The figure shows three views and two pictorial views of one solid part (mm, origin at its lowest corner). Answer the questions. Give positions to 0.01 mm unless a question says otherwise; leave off trailing zeros. Order: outer loops, then holes, each group sorted by start corner. A loop starts at its lowest first (then second) coordinate and runs counter-clockwise, first axis right, second up. Notation, with made-up numbers: (10.25, 27) - (59.25, 27) arc R20 ccw to (59.25, 54) - close; hole circle Ø11 at (16.5, -26.5). An arc over 180 degrees is marked (long way). Use a Markdown table: item, result. Add a question column.
1. Flat-ended cylindrical pins translate along their axes: P1, Ø6, axis at y = 4.5, z = 91.5, coming from the +X side; P2, Ø1.5, axis at y = 7.5, z = 113.5, coming from the -X side; P3, Ø1, axis at y = 4, z = 26, coming from the +X side; P4, Ø10, axis at x = 39, z = 59.5, coming from the -Y side. Find the tip coordinate at first contact, or state that the pin passes through.
2. Consider L1, parallel to X at y = 6, z = 110; L2, parallel to X at y = 1, z = 42; L3, parallel to Z at x = 35, y = 0.5. Determine where each line is inside the solid, lowest interval first.
3. A cutting plane is placed at C-C on y = 6.25. Determine the outline of the cut face in (x, z), and give its area (3 significant figures).
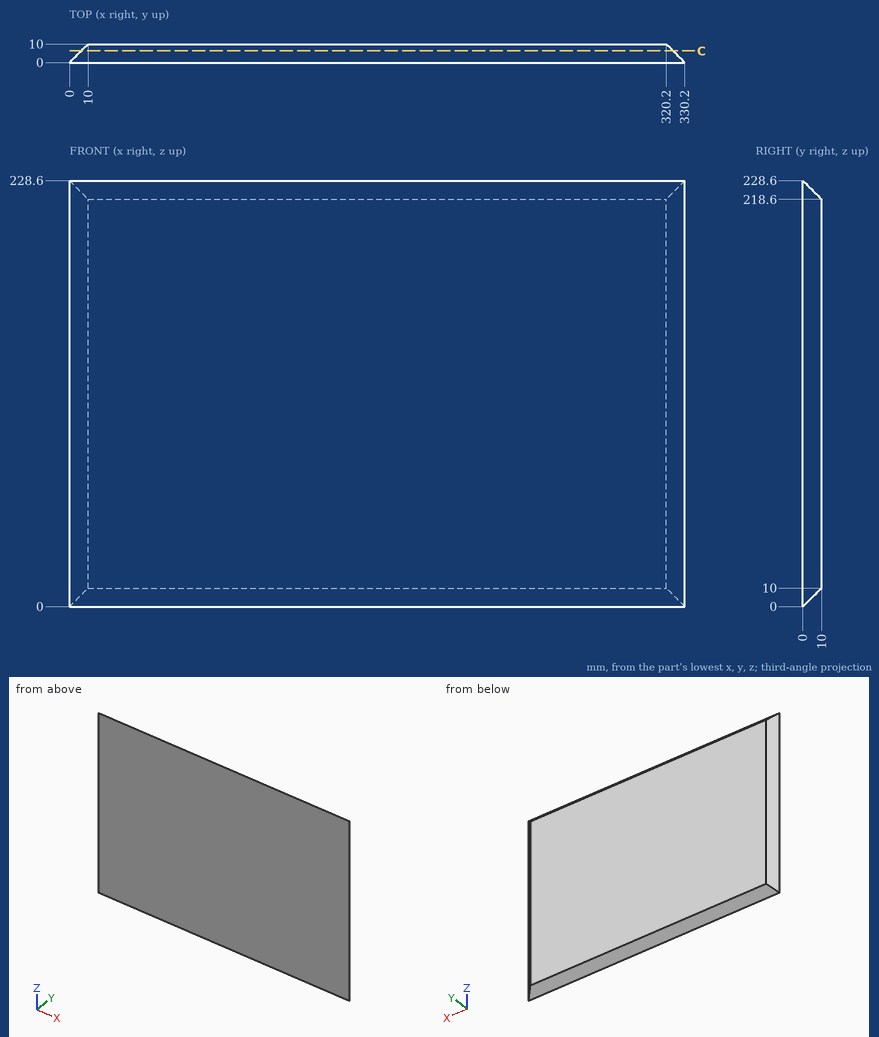
Output values:
| question | item | result |
|---|---|---|
| 1 | P1 | x = 328.7 |
| 1 | P2 | x = 6.75 |
| 1 | P3 | x = 326.7 |
| 1 | P4 | y = 0 |
| 2 | L1 | 6 to 324.2 |
| 2 | L2 | 1 to 329.2 |
| 2 | L3 | 0.5 to 228.1 |
| 3 | outline | (6.25, 6.25) - (323.95, 6.25) - (323.95, 222.35) - (6.25, 222.35) - close |
| 3 | area | 68,700 mm² |
